Autodesk Inventor part; units mm, degrees
ref_plane "YZ Plane" through (0, 0, 0) normal (1, 0, 0) x (0, 1, 0)
ref_plane "XZ Plane" through (0, 0, 0) normal (0, 1, 0) x (-1, 0, 0)
ref_plane "XY Plane" through (0, 0, 0) normal (0, 0, 1) x (1, 0, 0)
sketch "Sketch1" plane through (0, 0, 0) normal (0, 0, 1) x (1, 0, 0)
  line L0 (-46, -175) -> (46, -175)
  line L1 (46, -175) -> (46, 175)
  line L2 (46, 175) -> (-46, 175)
  line L3 (-46, 175) -> (-46, -175)
  line L4 (-46, -175) -> (46, 175) construction
  line L5 (46, -175) -> (-46, 175) construction
  point P0 (0, 0)
  dimension "d154" = 92
  dimension "d155" = 350
extrude "Plate5" add sketch "Sketch1" along normal blind 2
sketch "Sketch7" plane through (-44, -175, 0) normal (-1, 0, 0) x (0, -1, 0)
  line L0 (-350, 0) -> (0, 0)
  line L1 (0, 0) -> (0, 94)
  line L2 (0, 94) -> (-350, 94)
  line L3 (-350, 94) -> (-350, 0)
edge flange "Flange3" height 94 angle 90 thickness 2 bend radius 2.75 thickness toward (-1, 0, 0) relief round relief width 2 relief depth 1 edges at (-46, 0, 2) wall of the first edge with corners at (-44, 175, 0) (-44, -175, 0) (-44, -175, 94) (-44, 175, 94)
bend "Bend3"
corner "Corner3"
sketch "Sketch8" plane through (0, 0, 2) normal (0, 0, 1) x (1, 0, 0)
  line L0 (46, 175) -> (46, -175)
  line L1 (-41.25, 175) -> (46, 175)
  line L2 (31.375, 170) -> (-26.625, 170)
  line L3 (-26.625, 170) -> (-26.625, 112)
  line L4 (-26.625, 112) -> (31.375, 112)
  line L5 (31.375, 112) -> (31.375, 170)
  line L6 (31.375, 170) -> (-26.625, 112) construction
  line L7 (-26.625, 170) -> (31.375, 112) construction
  point P0 (0, 0)
  point P1 (2.375, 141)
  point P2 (2.375, 175)
  dimension "d167" = 58
  dimension "d168" = 58
  dimension "d169" = 5
extrude "Cut1" cut sketch "Sketch8" against normal blind 2
properties part number "PNS 752 FDS 1200 FLANGE 2_1600" material "Stainless Steel"
The model under review builds one solid part; all positions refer to its coordinate system, in mm. A direction names the side the tool comes from. Coordinates: 2 decimals unless noted, no trailing zeros. Write each loop counter-clockwise with the first axis right and the second up, starting at its lowest first coordinate (ties: lowest second). Pieces come first, ordered by that corner, then holes. Notation, with made-up numbers: (20.5, 18) - (39.5, 18) arc R19 cw to (39.5, 43) - close; hole circle Ø9 at (55, 36). An arc over 180 degrees is marked (long way). Answer as a JSON object with one key per item and string values. Group by question number.
1. Add section D-D (z = 30). Give the boundary of the cut face in (x, y).
2. Machinability: for faces 1 (the face through (-44, -2, 49)), 2 (the face through (2, -36, 0)), which of the approach directions +Z, -Z, +X, -X, +Y, -Y give a long, thin tool a straight path to every point of the face, cutting with its end or side? Answer none if there is none.
3. Add section A-A (y = 123). Give the boundary of the cut face in (x, z) (3 decimals), plus the area to 3 significant figures.
4. Add section C-C (y = -2.5). Give the boundary of the cut face in (x, z), plus the area to 3 significant figures.
5. Add section B-B (x = 12). Give the boundary of the cut face in (y, z).
6. Clearance check with flat-ended pins moving along their axes: pin 1 Ø4 at (y, z) = (114, 26) entering from +X; pin 2 Ø1 at (y, z) = (143, 1.5) entering from -X; pin 3 Ø1.5 at (x, y) = (32, 96.5) entering from +Z. State where each tip first meets the part, or that it passes through.
7. To check wall thickness, follow probe 1 along Z at (x, y) = (10, 4); probe 2 along X at (y, z) = (156.5, 15.5). State the ranges of each line that lie inside material, in increasing order.
Findings:
{
 "1": {"outline": "(-46, -175) - (-44, -175) - (-44, 175) - (-46, 175) - close"},
 "2": {"face 1": "+Z, +X, +Y, -Y", "face 2": "-Z, +X, -X, +Y, -Y"},
 "3": {"outline": "(-46, 4.75) arc R4.75 ccw to (-41.25, 0) - (-26.625, 0) - (-26.625, 2) - (-41.25, 2) arc R2.75 cw to (-44, 4.75) - (-44, 94) - (-46, 94) - close; (31.375, 0) - (46, 0) - (46, 2) - (31.375, 2) - close", "area": "249 mm²"},
 "4": {"outline": "(-46, 4.75) arc R4.75 ccw to (-41.25, 0) - (46, 0) - (46, 2) - (-41.25, 2) arc R2.75 cw to (-44, 4.75) - (-44, 94) - (-46, 94) - close", "area": "365 mm²"},
 "5": {"outline": "(-175, 0) - (112, 0) - (112, 2) - (-175, 2) - close; (170, 0) - (175, 0) - (175, 2) - (170, 2) - close"},
 "6": {"pin 1": "x = -44", "pin 2": "x = -45.12", "pin 3": "z = 2"},
 "7": {"probe 1": "0 to 2", "probe 2": "-46 to -44"}
}
